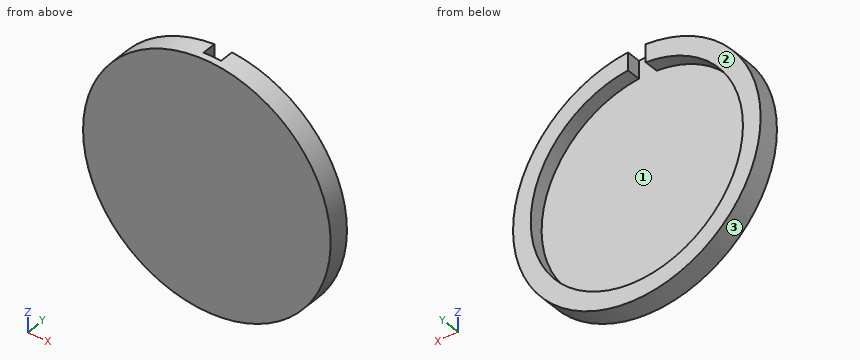
Autodesk Inventor part; units mm, degrees
ref_plane "YZ Plane" through (0, 0, 0) normal (1, 0, 0) x (0, 1, 0)
ref_plane "XZ Plane" through (0, 0, 0) normal (0, 1, 0) x (-1, 0, 0)
ref_plane "XY Plane" through (0, 0, 0) normal (0, 0, 1) x (1, 0, 0)
sketch "스케치1" plane through (0, 0, 0) normal (0, 1, 0) x (-1, 0, 0)
  circle A0 centre (0, 0) radius 70
  circle A1 centre (0, 0) radius 60
  line L0 (-59.7913, -5) -> (-69.8212, -5)
  line L1 (-59.7913, 5) -> (-69.8212, 5)
  dimension "d0" = 140
  dimension "d1" = 120
  dimension "d7" = 5
extrude "돌출1" add sketch "스케치1" along normal blind 12 contours A0 L0 A1 L1 | L1 A1 L0 A0
extrude "돌출2" add sketch "스케치1" along normal blind 4 contours A1
sketch "스케치2" plane through (0, 12, 0) normal (0, 1, 0) x (1, 0, 0)
  line L0 (5, -59.7913) -> (5, -69.8212)
  line L1 (-5, -59.7913) -> (-5, -69.8212)
  circle A0 centre (0, 0) radius 60
  circle A1 centre (0, 0) radius 70
  dimension "d8" = 10
  dimension "d9" = 5
extrude "돌출3" cut sketch "스케치2" against normal blind 8 contours L0 A1 L1 A0 picked at (3.8895, -63.1964)
properties part number "gps_case"
The listing builds one solid part. Answer for the finished solid, in the listing's coordinates (mm). Face numbers are marked on the shaded views. Give positions to 0.01 mm unless a question says otherwise; leave off trailing zeros. Order: outer loops, then holes, each group sorted by start corner. A loop starts at its lowest first (then second) coordinate and runs counter-clockwise, first axis right, second up. Notation, with made-up numbers: (55.5, 74.25) - (111.5, 74.25) arc R13 ccw to (111.5, 81.25) - close; hole circle Ø3 at (46.25, -20.5). An arc over 180 degrees is marked (long way). Use one line per item in the form item = value. Start each with the question number.
(1) A cutting plane is placed at A-A, the plane z = 0. Write down the section's boundary in (x, y), then the cut area to 3 significant figures.
(2) Flat-ended cylindrical pins translate along their axes: pin 1 Ø1 at (x, y) = (14, 8.5) entering from -Z; pin 2 Ø4 at (y, z) = (6, 64) entering from -X; pin 3 Ø1 at (y, z) = (7.5, -36) entering from +X. Find the tip coordinate at first contact, or state that the pin passes through.
(3) A cutting plane is placed at D-D, the plane x = 0. Write down the section's boundary in (y, z), then the cut area to 3 significant figures.
(4) Consider line 1 (X direction, y = 7.5, z = 0); line 2 (Y direction, x = 1.5, z = 56); line 3 (Z direction, x = 13.5, y = 4.5). Determine where each line is inside the solid, lowest interval first. Write a range as from..to.
(5) A cutting plane is placed at C-C, the plane y = 7.5. Write down the section's boundary in (x, z), then the cut area to 3 significant figures.
(6) The mould has two halves that part along Z. Classify the marked faces 1, 2 and 3: released by +Z, released by -Z, zero draft, split by the parting line, or undercut.
(7) A cutting plane is placed at B-B, the plane x = 36. Write down the section's boundary in (y, z), then the cut area to 3 significant figures.
Ans:
q1.outline = (-70, 0) - (70, 0) - (70, 12) - (60, 12) - (60, 4) - (-60, 4) - (-60, 12) - (-70, 12) - close
q1.area = 720 mm^2
q2.pin_1 = -68.69
q2.pin_2 = -32.5
q2.pin_3 = 60.33
q3.outline = (0, -70) - (12, -70) - (12, -60) - (4, -60) - (4, 70) - (0, 70) - close
q3.area = 640 mm^2
q4.line_1 = -70..-60, 60..70
q4.line_2 = 0..4
q4.line_3 = -68.69..-58.46, 58.46..68.69
q5.outline = (-5, 59.79) - (-5, 69.82) arc R70 ccw (long way) to (5, 69.82) - (5, 59.79) arc R60 cw (long way) to start
q5.area = 3,980 mm^2
q6.face_1 = undercut
q6.face_2 = zero draft
q6.face_3 = split by the parting line
q7.outline = (0, -60.03) - (12, -60.03) - (12, -48) - (4, -48) - (4, 48) - (12, 48) - (12, 60.03) - (0, 60.03) - close
q7.area = 673 mm^2
